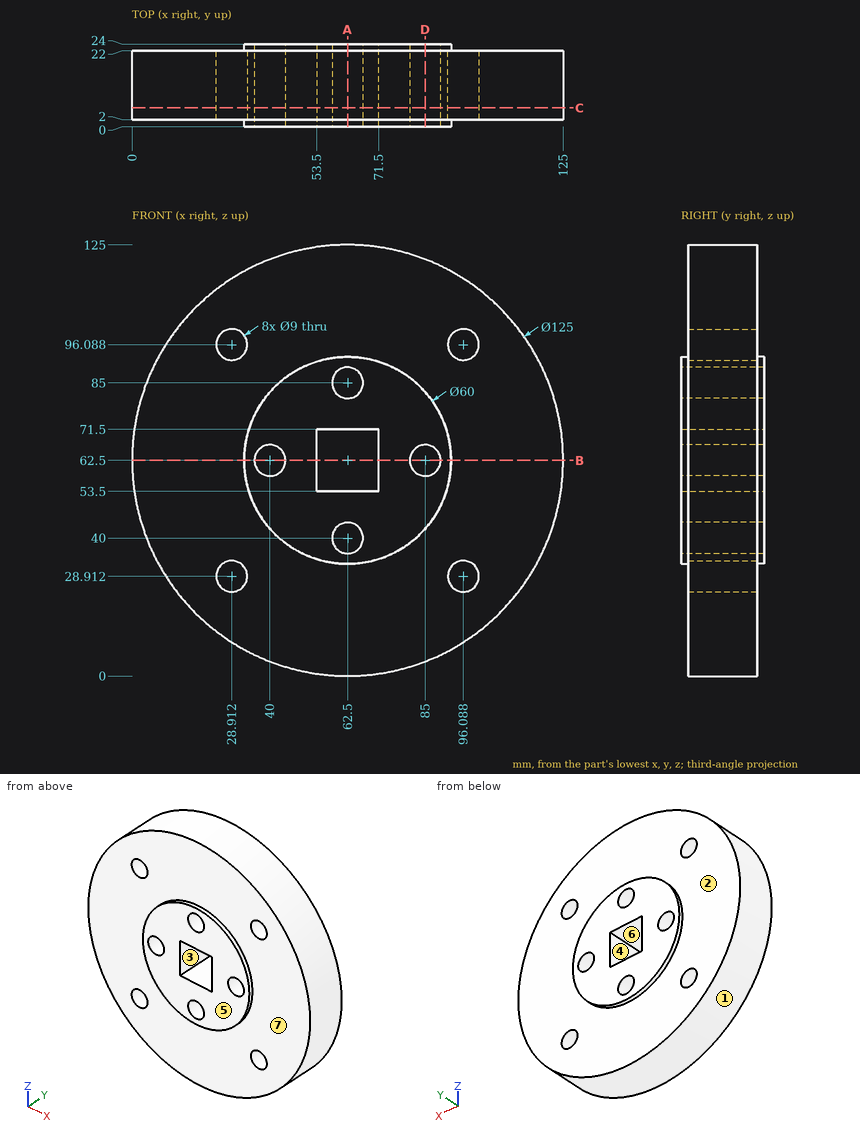
Verification items for this drawing (mm, ordinates from the low corner). A direction names the side the tool comes from. Coordinates: 2 decimals unless noted, no trailing zeros. Order: outer loops, then holes, each group sorted by start corner. A loop starts at its lowest first (then second) coordinate and runs counter-clockwise, first axis right, second up. Notation, with made-up numbers: (56.25, 4.5) - (75.25, 4.5) arc R25 ccw to (75.25, 28.5) - close; hole circle Ø9 at (52.5, 4). An arc over 180 degrees is marked (long way). Answer as a JSON object with one key per item and string values. Group by question number.
Item 1: Tool access check on the marked faces 5, 6 and 7. Record the directions out of +Z, -Z, +X, -X, +Y, -Y that give a thin tool (end or side, any length) a straight path to the whole face; none if there is none.
Item 2: Sectioned sample at B-B, the plane z = 62.5. Record the cut outline in (x, y).
Item 3: Depth check by flat-ended pin: pin 1 Ø10 at (y, z) = (20.5, 105) entering from +X; pin 2 Ø7 at (x, z) = (40, 62.5) entering from -Y; pin 3 Ø4 at (x, y) = (31.5, 17) entering from -Z (1 decimal); pin 4 Ø10.5 at (x, z) = (28.91, 28.91) entering from +Y. Enter the tip coordinate at first touch or a pass-through.
Item 4: Scan lines: probe 1 along Z at (x, y) = (62.5, 17.5); probe 2 along X at (y, z) = (9.5, 61); probe 3 along Y at (x, z) = (96, 43). Record each from-to range of solid material in increasing order.
Item 5: Draft check along Z on the marked faces 1, 2, 3 and 4. Enter one of: +Z half, -Z half, draft (parallel to the pull), parting line (faces both ways), or undercut.
Item 6: Sectioned sample at D-D, the plane x = 85. Record the cut outline in (y, z), and give its area (4 significant figures).
Item 7: Sectioned sample at C-C, the plane y = 5.5. Give the number of separate pieces and of enclosed holes in the cut face, and give its area (3 significant figures).
Item 8: Sectioned sample at A-A, the plane x = 62.5. Record the cut outline in (y, z), and give its area (3 significant figures).
Resolved:
{
 "1": {"face 5": "+Z, -Z, +X, -X, -Y", "face 6": "+Y, -Y", "face 7": "-Y"},
 "2": {"outline": "(0, 2) - (32.5, 2) - (32.5, 0) - (35.5, 0) - (35.5, 24) - (32.5, 24) - (32.5, 22) - (0, 22) - close; (44.5, 0) - (53.5, 0) - (53.5, 24) - (44.5, 24) - close; (71.5, 0) - (80.5, 0) - (80.5, 24) - (71.5, 24) - close; (89.5, 0) - (92.5, 0) - (92.5, 2) - (125, 2) - (125, 22) - (92.5, 22) - (92.5, 24) - (89.5, 24) - close"},
 "3": {"pin 1": "x = 112.5", "pin 2": "through", "pin 3": "z = 7.1", "pin 4": "y = 22"},
 "4": {"probe 1": "0 to 35.5, 44.5 to 53.5, 71.5 to 80.5, 89.5 to 125", "probe 2": "0.02 to 35.76, 44.24 to 53.5, 71.5 to 80.76, 89.24 to 124.98", "probe 3": "2 to 22"},
 "5": {"face 1": "parting line", "face 2": "draft", "face 3": "undercut", "face 4": "undercut"},
 "6": {"outline": "(0, 42.66) - (2, 42.66) - (2, 4.19) - (22, 4.19) - (22, 42.66) - (24, 42.66) - (24, 58) - (0, 58) - close; (0, 67) - (24, 67) - (24, 82.34) - (22, 82.34) - (22, 120.81) - (2, 120.81) - (2, 82.34) - (0, 82.34) - close", "area": "2,275 mm^2"},
 "7": {"separate pieces": "1", "enclosed holes": "9", "area": "11,400 mm^2"},
 "8": {"outline": "(0, 32.5) - (2, 32.5) - (2, 0) - (22, 0) - (22, 32.5) - (24, 32.5) - (24, 35.5) - (0, 35.5) - close; (0, 44.5) - (24, 44.5) - (24, 53.5) - (0, 53.5) - close; (0, 71.5) - (24, 71.5) - (24, 80.5) - (0, 80.5) - close; (0, 89.5) - (24, 89.5) - (24, 92.5) - (22, 92.5) - (22, 125) - (2, 125) - (2, 92.5) - (0, 92.5) - close", "area": "1,880 mm^2"}
}
